The listing builds one solid part. Answer for the finished solid, in the listing's coordinates (mm). A direction names the side the tool comes from. Coordinates: 2 decimals unless noted, no trailing zeros. Write each loop counter-clockwise with the first axis right and the second up, starting at its lowest first coordinate (ties: lowest second). Pieces come first, ordered by that corner, then holes.
from build123d import *

# Parameters (mm, degrees)
SKETCH1_R               = 9
SKETCH1_R_2             = 3.05
BOSS_EXTRUDE1_DEPTH     = 8
BOSS_EXTRUDE2_START     = 7
SKETCH1_3_R             = 9
BOSS_EXTRUDE2_DEPTH     = 7
BOSS_EXTRUDE3_START     = -12
BOSS_EXTRUDE3_OUTLINE_R = 9
BOSS_EXTRUDE3_DEPTH     = 12
SKETCH3_3_R             = 9
SKETCH3_3_R_2           = 5.05
BOSS_EXTRUDE4_DEPTH     = 10


# Read off the part's stored shape, not the designer's step: Boss-Extrude3
with BuildPart() as part:
    # Sketch1 → Boss-Extrude1 (new body)
    with BuildSketch(Plane.XY):
        Circle(SKETCH1_R)
        Circle(SKETCH1_R_2, mode=Mode.SUBTRACT)
    extrude(amount=-BOSS_EXTRUDE1_DEPTH)

    # Sketch1_3 → Boss-Extrude2 (add)
    with BuildSketch(Plane.XY.offset(BOSS_EXTRUDE2_START)):
        Circle(SKETCH1_3_R)
        with BuildLine():
            Line((2.5, 1.747140521), (2.5, -1.747140521))
            ThreePointArc((2.5, -1.747140521), (-3.05, 0), (2.5, 1.747140521))
        make_face(mode=Mode.SUBTRACT)
    extrude(amount=-BOSS_EXTRUDE2_DEPTH)



with BuildPart() as body_2:
    # Boss-Extrude3 outline → Boss-Extrude3 (new body)
    with BuildSketch(Plane(origin=(0, 0, 16.5), x_dir=(-1, 0, 0), z_dir=(0, 0, -1)).offset(BOSS_EXTRUDE3_START)):
        with Locations((0, -0.074857464)):
            Circle(BOSS_EXTRUDE3_OUTLINE_R)
        with BuildLine():
            ThreePointArc((-4.000061363, 3.082532902), (5.05, 0), (-4.000061363, -3.082532902))
            Line((-4.000061363, -3.082532902), (-4.000061363, 0))
            Line((-4.000061363, 0), (-4.016547732, 2.977808644))
            ThreePointArc((-4.016547732, 2.977808644), (-4.008319792, 2.98887478), (-4.000061363, 2.999918181))
            Line((-4.000061363, 2.999918181), (-4.000061363, 3.082532902))
        make_face(mode=Mode.SUBTRACT)
    extrude(amount=BOSS_EXTRUDE3_DEPTH)


with BuildPart() as part_1:
    add(part.part)

    add(body_2.part)  # Boss-Extrude4 merges body 2
    # Sketch3_3 → Boss-Extrude4 (add)
    with BuildSketch(Plane(origin=(0, 0, 16.5), x_dir=(-1, 0, 0), z_dir=(0, 0, -1))):
        with Locations(Location((0, -0.074857464, 0), (0, 0, 0.238279395))):
            Circle(SKETCH3_3_R)
        with Locations(Location((0, 0, 0), (0, 0, 217.618616))):
            Circle(SKETCH3_3_R_2, mode=Mode.SUBTRACT)
    extrude(amount=BOSS_EXTRUDE4_DEPTH)


solid = part_1.part
1. A tool of negligible diameter and unlimited length cuts with its end or side. For faces 5 (the cylindrical face through (-8.584, 2.63, 17.654)), 6 (the flat face through (2.5, 0, 4)), 7 (the flat face through (0, -4, -8)), from which of +Z, -Z, +X, -X, +Y, -Y can it reach the whole face along a straight path? Write none if from no direction.
Results found:
face 5: +Z
face 6: +Z, -Z
face 7: -Z, +X, -X, +Y, -Y
2. Section C-C on z = -5 is taken. Give the vertices of the cut face in (x, y), then the cut area to 3 significant figures.
Results found:
outline: circle Ø18 at (0, 0); hole circle Ø6.1 at (0, 0)
area: 225 mm2
3. Find the intervals of material crossed by L1, parallel to Y at x = 0, z = 11.5; L2, parallel to X at y = 0, z = 12.75; L3, parallel to X at y = 0, z = 2.25, in increasing order.
Results found:
L1: y = -9.07 to -5.05, 5.05 to 8.93
L2: x = -9 to -5.05, 5.05 to 9
L3: x = -9 to -3.05, 2.5 to 9
4. Section D-D on y = 7.75 is taken. Give the vertices of the cut face in (x, z), then the cut area to 3 significant figures.
Results found:
outline: (-4.58, -8) - (4.58, -8) - (4.58, 7) - (4.45, 7) - (4.45, 28.5) - (-4.45, 28.5) - (-4.45, 7) - (-4.58, 7) - close
area: 328 mm2
5. Flat-ended cylindrical pins translate along their axes: P1, Ø2, axis at y = -5, z = 22.5, coming from the -X side; P2, Ø1.5, axis at y = 6.5, z = 8.5, coming from the +X side; P3, Ø3.5, axis at x = 0, y = 0, coming from the -Z side; P4, Ø3, axis at x = 3, z = 9.5, coming from the -Y side. Find the tip coordinate at first contact, or state that the pin passes through.
Results found:
P1: stops at x = -8.1
P2: stops at x = 6.86
P3: passes through
P4: stops at y = -8.95
6. Section A-A on x = 0 is taken. Give the vertices of the cut face in (y, z), then the cut area to 3 significant figures.
Results found:
outline: (-9.07, 6.5) - (-9, 6.5) - (-9, -8) - (-3.05, -8) - (-3.05, 7) - (-5.05, 7) - (-5.05, 28.5) - (-9.07, 28.5) - close; (3.05, -8) - (9, -8) - (9, 7) - (8.93, 7) - (8.93, 28.5) - (5.05, 28.5) - (5.05, 7) - (3.05, 7) - close
area: 348 mm2
7. For a pull along X with two mould halves and no side action, classify faces 1 (the flat face through (4.4, 0, 16.5)), 2 (the flat face through (-4, -4, 28.5)), 3 (the flat face through (3, 0, 7)), 4 (the cylindrical face through (-1.172, 8.923, -0.395)) as pulls with the +X half, pulls with the -X half, needs draft (parallel to the pull), parting line crosses it, or undercut.
Results found:
face 1: undercut
face 2: needs draft
face 3: undercut
face 4: parting line crosses it
